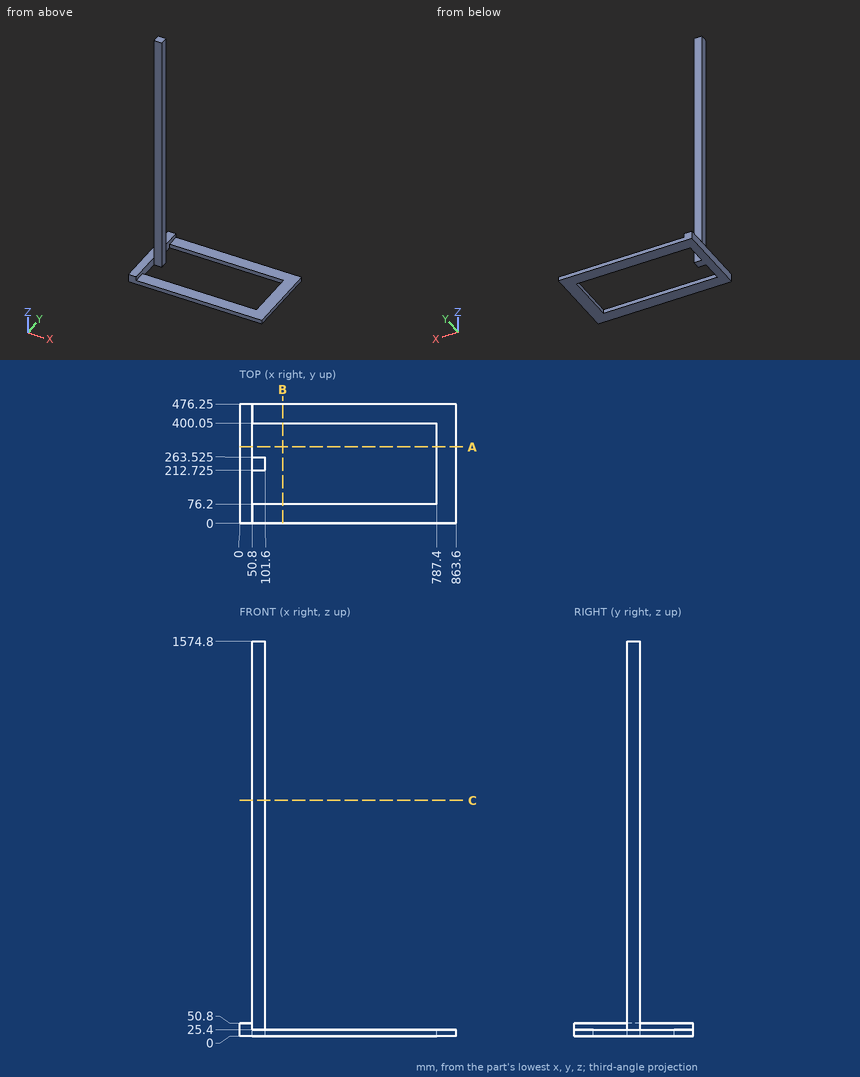
Answer from the drawing. Dimensions are ordinates in mm from the lowest x, y and z of the part. Coordinates: 2 decimals unless noted, no trailing zeros. Loops run counter-clockwise (first coordinate to the right, second up) from the corner with the lowest first, then second, coordinate; pieces in that order, holes last.
1) Flat-ended cylindrical pins translate along their axes: pin 1 (15 mm diameter, centred on x = 86, z = 1126.5, fed in from -Y) (3 decimals); pin 2 (15 mm diameter, centred on x = 22.5, y = 333, fed in from +Z); pin 3 (15 mm diameter, centred on x = 72, z = 787.5, fed in from +Y) (3 decimals). Find the tip coordinate at first contact, or state that the pin passes through.
Results:
pin 1: stops at y = 212.725
pin 2: stops at z = 50.8
pin 3: stops at y = 263.525
2) Section C-C (z = 940.5) is taken. Give the vertices of the cut face in (x, y) (3 decimals).
Results:
outline: (50.8, 212.725) - (101.6, 212.725) - (101.6, 263.525) - (50.8, 263.525) - close
3) Section A-A (y = 305) is taken. Give the vertices of the cut face in (x, z).
Results:
outline: (0, 0) - (50.8, 0) - (50.8, 50.8) - (0, 50.8) - close; (787.4, 0) - (863.6, 0) - (863.6, 25.4) - (787.4, 25.4) - close
4) Section B-B (x = 172) is taken. Give the vertices of the cut face in (y, z), plus the area to 3 significant figures.
Results:
outline: (0, 0) - (76.2, 0) - (76.2, 25.4) - (0, 25.4) - close; (400.05, 0) - (476.25, 0) - (476.25, 25.4) - (400.05, 25.4) - close
area: 3,870 mm2
5) Consider probe 1 along X at (y, z) = (260.5, 1117); probe 2 along Y at (x, z) = (74, 957.5) (3 decimals); probe 3 along Z at (x, y) = (710, 40.5). Determine where each line is inside the solid, lowest interval first.
Results:
probe 1: x = 50.8 to 101.6
probe 2: y = 212.725 to 263.525
probe 3: z = 0 to 25.4
